Can you work these out from the drawing? Everything is in mm from the part's minimum corner. Round coordinates to 2 decimals unless told otherwise and drop trailing zeros. Loops run counter-clockwise (first coordinate to the right, second up) from the corner with the lowest first, then second, coordinate; pieces in that order, holes last. Notation, with made-up numbers: (-20, 42.5) -> (32, 42.5) arc R19 ccw to (32, 67.5) -> close; hole circle Ø9 at (-12.75, -38.75). An arc over 180 degrees is marked (long way). Use CSV: the item, a comma, the result in double quotes. Start each with the question number.
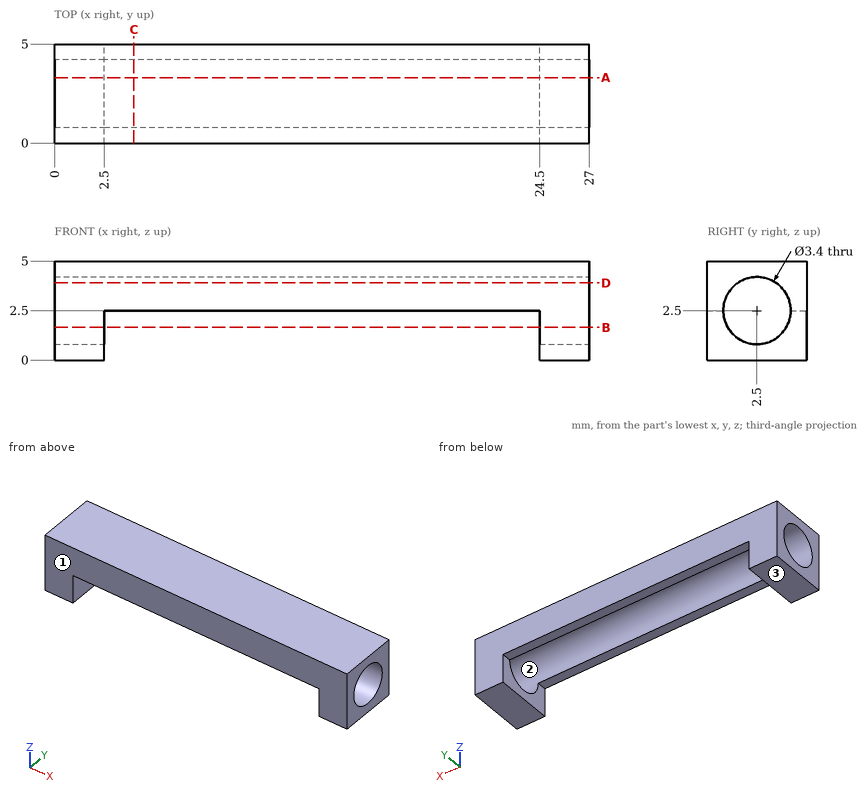
1. If I drill on L1, parallel to X at y = 0.35, z = 0.95; L2, parallel to Z at x = 5.5, y = 4.3; L3, parallel to Y at x = 12.75, z = 3.85, over which ranges is the centre line in solid material (lowest first)?
2. We'd pull the mould along Y, two halves only. Please class the marked faces 1, 2 and 3: pulls with the +Y half, pulls with the -Y half, needs draft (parallel to the pull), parting line crosses it, or undercut.
3. Suppose I cut it at B-B (z = 1.65). List the corners of the cut face in (x, y) for me, then the cut area to 3 significant figures.
4. Suppose I cut it at A-A (y = 3.3). List the corners of the cut face in (x, z) for me, then the cut area to 3 significant figures.
5. Suppose I cut it at C-C (x = 4). List the corners of the cut face in (y, z) for me, then the cut area to 3 significant figures.
6. Suppose I cut it at D-D (z = 3.9). List the corners of the cut face in (x, y) for me.
7. Will these pins go through, and if not, where does the flat tip stop? pin 1 (0.9 mm diameter, centred on x = 16.5, y = 0.5, fed in from -Z); pin 2 (3 mm diameter, centred on y = 2.5, z = 2.5, fed in from +X).
Geometry check:
1,L1,"x = 0 to 2.5, 24.5 to 27"
1,L2,"z = 2.5 to 5"
1,L3,"y = 0 to 1.47, 3.53 to 5"
2,face 1,"pulls with the -Y half"
2,face 2,"undercut"
2,face 3,"needs draft"
3,outline,"(0, 0) -> (2.5, 0) -> (2.5, 1.03) -> (0, 1.03) -> close; (0, 3.97) -> (2.5, 3.97) -> (2.5, 5) -> (0, 5) -> close; (24.5, 0) -> (27, 0) -> (27, 1.03) -> (24.5, 1.03) -> close; (24.5, 3.97) -> (27, 3.97) -> (27, 5) -> (24.5, 5) -> close"
3,area,"10.3 mm²"
4,outline,"(0, 0) -> (2.5, 0) -> (2.5, 1) -> (0, 1) -> close; (0, 4) -> (27, 4) -> (27, 5) -> (0, 5) -> close; (24.5, 0) -> (27, 0) -> (27, 1) -> (24.5, 1) -> close"
4,area,"32.0 mm²"
5,outline,"(0, 2.5) -> (0.8, 2.5) arc R1.7 cw to (4.2, 2.5) -> (5, 2.5) -> (5, 5) -> (0, 5) -> close"
5,area,"7.96 mm²"
6,outline,"(0, 0) -> (27, 0) -> (27, 1.54) -> (0, 1.54) -> close; (0, 3.46) -> (27, 3.46) -> (27, 5) -> (0, 5) -> close"
7,pin 1,"stops at z = 2.5"
7,pin 2,"passes through"
